from build123d import *

# Parameters (mm, degrees)
BOSS_EXTRUDE1_DEPTH = 25.4
FILLET1_R           = 12.7
SKETCH2_R           = 3.175
CUT_EXTRUDE1_DEPTH  = 3.54
SKETCH3_R           = 2.4765
CUT_EXTRUDE2_DEPTH  = 3.512939161


with BuildPart() as part:
    # Sketch1 → Boss-Extrude1 (new body)
    with BuildSketch(Plane.XY):
        Polygon((-12.7, -12.7), (-12.7, 12.7), (4.47675, 12.7), (4.47675, 10.187060839), (-10.16, 10.187060839), (-10.16, -12.7), align=None)
    extrude(amount=BOSS_EXTRUDE1_DEPTH)

    # Fillet1
    fillet1_edges = [part.edges().sort_by_distance(p)[0] for p in [
        (-11.43, -12.7, 0),
    ]]
    fillet(fillet1_edges, radius=FILLET1_R)

    # Sketch2 → Cut-Extrude1 (cut, through all)
    with BuildSketch(Plane(origin=(-10.16, 0, 0), x_dir=(0, 0, -1), z_dir=(1, 0, 0))):
        with Locations((-10.45493597, -2.24506403)):
            Circle(SKETCH2_R)
    extrude(amount=-CUT_EXTRUDE1_DEPTH, mode=Mode.SUBTRACT)

    # Sketch3 → Cut-Extrude2 (cut, through all)
    with BuildSketch(Plane.XZ.offset(-10.187060839)):
        with Locations((-3.175, 19.05)):
            Circle(SKETCH3_R)
        with Locations((-3.175, 6.35)):
            Circle(SKETCH3_R)
    extrude(amount=-CUT_EXTRUDE2_DEPTH, mode=Mode.SUBTRACT)


solid = part.part
Design review of the part built by this model. Coordinates are the model's own, in mm. A direction names the side the tool comes from. Give positions to 0.01 mm unless a question says otherwise; leave off trailing zeros. Order: outer loops, then holes, each group sorted by start corner. A loop starts at its lowest first (then second) coordinate and runs counter-clockwise, first axis right, second up. Notation, with made-up numbers: (51, 10) - (104, 10) arc R20 cw to (104, 19) - close; hole circle Ø3 at (51.5, 12). An arc over 180 degrees is marked (long way). Write item = value, one per line. Start each with the question number.
Q1. We need section C-C on y = 6.75. State the section outline as (x, z) points.
Q2. Tool access review of faces 1 (the face through (-7, 12, 0)), 2 (the face through (-10.16, 1, 13)): name each direction out of +Z, -Z, +X, -X, +Y, -Y from which nothing blocks a thin tool from reaching the whole face with its end or side.
Q3. We need section D-D on z = 2.75. State the section outline as (x, y) points.
Q4. Clearance check with flat-ended pins moving along their axes: pin 1 Ø6 at (x, z) = (2.5, 6.5) entering from -Y; pin 2 Ø10 at (x, y) = (-8.5, 7.5) entering from -Z; pin 3 Ø1 at (x, y) = (-10, -6) entering from -Z; pin 4 Ø7 at (y, z) = (0, 13.5) entering from +X. State where each tip first meets the part, or that it passes through.
Q5. We need section B-B on x = -4. State the section outline as (y, z) points.
Q6. Mouldability with a two-part tool opening along Z and no side actions: class faces 3 (the face through (-3, 10.187, 13)), 4 (the face through (-2.032, 11.426, 16.853)), 5 (the face through (-11.45, -9.08, 3.82)) as released by +Z, released by -Z, zero draft, split by the parting line, or undercut.
Q7. We need section A-A on z = 19.05. State the section outline as (x, y) points.
Q8. To check wall thickness, follow L1, parallel to Y at x = -0.5, z = 22.25; L2, parallel to X at y = 0.75, z = 6.25; L3, parallel to Y at x = -11.25, z = 11.5. State the ranges of each line that lie inside material, in increasing order. Write a range as from..to.
Working result:
q1.outline = (-12.7, 0) - (-10.16, 0) - (-10.16, 25.4) - (-12.7, 25.4) - close
q2.face_1 = -Z, +X, -X, +Y, -Y
q2.face_2 = +Z, -Z, +X, -Y
q3.outline = (-12.7, -7.89) - (-10.16, -7.89) - (-10.16, 10.19) - (4.48, 10.19) - (4.48, 12.7) - (-12.7, 12.7) - close
q4.pin_1 = 10.19
q4.pin_2 = 0
q4.pin_3 = 1.27
q4.pin_4 = -10.16
q5.outline = (10.19, 0) - (12.7, 0) - (12.7, 4.01) - (10.19, 4.01) - close; (10.19, 8.69) - (12.7, 8.69) - (12.7, 16.71) - (10.19, 16.71) - close; (10.19, 21.39) - (12.7, 21.39) - (12.7, 25.4) - (10.19, 25.4) - close
q6.face_3 = zero draft
q6.face_4 = undercut
q6.face_5 = released by -Z
q7.outline = (-12.7, -12.7) - (-10.16, -12.7) - (-10.16, 10.19) - (-5.65, 10.19) - (-5.65, 12.7) - (-12.7, 12.7) - close; (-0.7, 10.19) - (4.48, 10.19) - (4.48, 12.7) - (-0.7, 12.7) - close
q8.L1 = 10.19..12.7
q8.L2 = -12.7..-10.16
q8.L3 = -12.64..-5.24, 0.75..12.7
